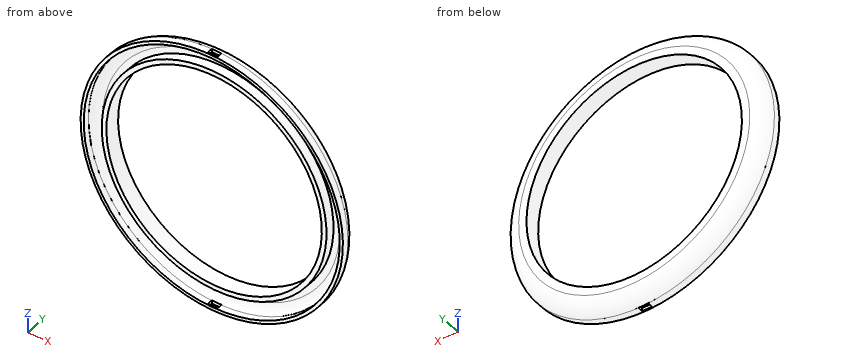
```python
from build123d import *

# Parameters (mm, degrees)
SKETCH_2_W               = 3.1
SKETCH_2_H               = 1.6
CUT_EXTRUDE_1_DEPTH      = 5
PATTERN_CIRCULAR_2_COUNT = 2


with BuildPart() as part:
    # Эскиз1 → Повернуть1 (revolve)
    with BuildSketch(Plane(origin=(0, 0, 0), x_dir=(0, 0, -1), z_dir=(1, 0, 0))):
        with BuildLine():
            Line((36, 0), (36, 3))
            Line((36, 3), (38, 3))
            ThreePointArc((38, 3), (39.809588321, 2.464382482), (41, 1))
            Line((41, 1), (41, -1))
            Line((41, -1), (42, -1))
            Line((42, -1), (42, 1.115227568))
            ThreePointArc((42, 1.115227568), (40.165890745, 3.914666233), (37, 5))
            Line((37, 5), (34.5, 5))
            Line((34.5, 5), (34.5, 0))
            Line((34.5, 0), (36, 0))
        make_face()
    revolve(axis=Axis((0, 0, 0), (0, 1, 0)))

    # Эскиз2 → Вырез-Вытянуть1 (cut)
    with BuildSketch(Plane(origin=(0, 0, -42), x_dir=(-1, 0, 0), z_dir=(0, 0, -1))):
        with Locations((0, 0.3)):
            Rectangle(SKETCH_2_W, SKETCH_2_H)
    cut_extrude_1 = extrude(amount=-CUT_EXTRUDE_1_DEPTH, mode=Mode.SUBTRACT)

    # Круговой массив2: Вырез-Вытянуть1 ×2 about axis
    pattern_circular_2_axis = Axis((0, 0, 0), (0, -1, 0))
    for i in range(1, PATTERN_CIRCULAR_2_COUNT):
        add(cut_extrude_1.rotate(pattern_circular_2_axis, i * 360 / PATTERN_CIRCULAR_2_COUNT), mode=Mode.SUBTRACT)


solid = part.part
```
CAD build for the part. Positions are in the model's coordinates, mm. Round coordinates to 2 decimals unless told otherwise and drop trailing zeros. Order: outer loops, then holes, each group sorted by start corner. A loop starts at its lowest first (then second) coordinate and runs counter-clockwise, first axis right, second up.
Q1. Slice it at B-B (x = 0). State how many separate pieces and enclosed holes the cut face has, and give its area (3 significant figures).
Q2. Slice it at A-A (z = 0). Write the cut outline in (x, y).
Q3. Slice it at C-C (y = 3.95). Write the cut outline in (x, z), and give its area (3 significant figures).
Q4. Drop flat-ended pins along their axis: pin 1 (3 mm diameter, centred on x = 14, y = 0, fed in from +Z); pin 2 (0.8 mm diameter, centred on x = 0, z = -41.5, fed in from +Y); pin 3 (8 mm diameter, centred on x = 29.5, z = -2.5, fed in from +Y); pin 4 (1.1 mm diameter, centred on x = 0.5, z = 41.5, fed in from +Y). Give the stop position or say it passes through.
Q5. Wall check: L1, parallel to X at y = 0.15, z = 0; L2, parallel to X at y = 2.6, z = -11; L3, parallel to Z at x = 0, y = -0.6. Give the ranges that are in metal, low to high.
Results below:
1. separate pieces: 4
1. enclosed holes: 0
1. area: 37.0 mm2
2. outline: (-42, -1) - (-41, -1) - (-41, 1) arc R3.19 cw to (-38, 3) - (-36, 3) - (-36, 0) - (-34.5, 0) - (-34.5, 5) - (-37, 5) arc R5.16 ccw to (-42, 1.12) - close; (34.5, 0) - (36, 0) - (36, 3) - (38, 3) arc R3.19 cw to (41, 1) - (41, -1) - (42, -1) - (42, 1.12) arc R5.16 ccw to (37, 5) - (34.5, 5) - close
3. outline: circle Ø80.24 at (0, 0); hole circle Ø69 at (0, 0)
3. area: 1,320 mm2
4. pin 1: stops at z = 40.1
4. pin 2: stops at y = 2.97
4. pin 3: passes through
4. pin 4: stops at y = 3.16
5. L1: x = -42 to -41, -36 to -34.5, 34.5 to 36, 41 to 42
5. L2: x = -39.87 to -38.03, -34.28 to -32.7, 32.7 to 34.28, 38.03 to 39.87
5. L3: z = -42 to -41, 41 to 42
